Geometry: final body of the model. Coordinates: model frame, mm. Give positions to 0.01 mm unless a question says otherwise; leave off trailing zeros. Loops run counter-clockwise (first coordinate to the right, second up) from the corner with the lowest first, then second, coordinate; pieces in that order, holes last. Notation, with made-up numbers: (13, 65.25) - (55, 65.25) arc R25 ccw to (55, 87.25) - close; hole circle Ø7 at (-1, 60). An arc over 180 degrees is marked (long way). Answer in a Markdown table with one row per item.
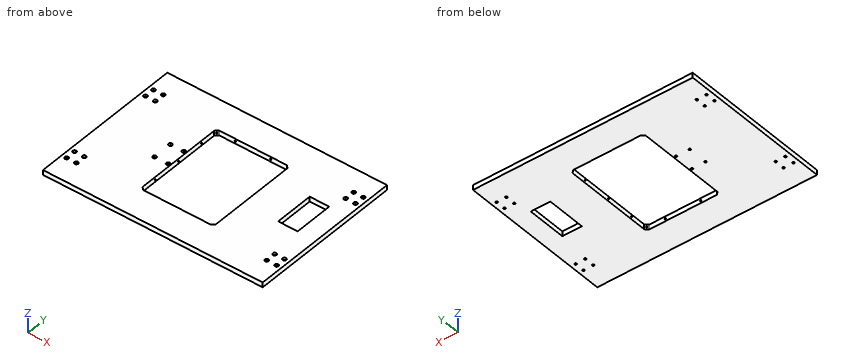
from build123d import *

# Parameters (mm, degrees)
SKETCH1_W                                            = 900
SKETCH1_H                                            = 630
BOSS_EXTRUDE1_DEPTH                                  = 20
SKETCH2_W                                            = 300
SKETCH2_H                                            = 385
CUT_EXTRUDE1_DEPTH                                   = 550.65898519
CHAMFER1_SIZE                                        = 11
FILLET1_R                                            = 3
M6_TAPPED_HOLE2_AT_2_COUNT                           = 2
M6_TAPPED_HOLE2_AT_2_PITCH                           = 117.5
CBORE_FOR_M8_HEXAGON_SOCKET_HEAD_CAP_SCR_D           = 8.4
CBORE_FOR_M8_HEXAGON_SOCKET_HEAD_CAP_SCR_CBORE_D     = 15
CBORE_FOR_M8_HEXAGON_SOCKET_HEAD_CAP_SCR_CBORE_DEPTH = 9
SKETCH13_W                                           = 80
SKETCH13_H                                           = 160
CUT_EXTRUDE3_DEPTH                                   = 550.65898519


with BuildPart() as part:
    # Sketch1 → Boss-Extrude1 (new body)
    with BuildSketch(Plane.XY):
        Rectangle(SKETCH1_W, SKETCH1_H)
    extrude(amount=BOSS_EXTRUDE1_DEPTH)

    # Sketch2 → Cut-Extrude1 (cut, through all)
    with BuildSketch(Plane.XY.offset(20)):
        Rectangle(SKETCH2_W, SKETCH2_H)
    extrude(amount=-CUT_EXTRUDE1_DEPTH, mode=Mode.SUBTRACT)

    # Chamfer1
    chamfer1_edges = [part.edges().sort_by_distance(p)[0] for p in [
        (-150, -192.5, 10),
        (-150, 192.5, 10),
        (150, 192.5, 10),
        (150, -192.5, 10),
    ]]
    chamfer(chamfer1_edges, length=CHAMFER1_SIZE)

    # Sketch4 → M6 Tapped Hole1 (revolve, cut)
    with BuildSketch(Plane(origin=(-144.5, 187, 10), x_dir=(0.7071067811865441, 0.7071067811865509, 0), z_dir=(0, 0, 1))):
        Polygon((0, 0), (0, 31.502151548), (2.5, 30), (2.5, 0), align=None)
    m6_tapped_hole1 = revolve(axis=Axis((-140.009871939, 182.509871939, 10), (-0.7071067811865509, 0.7071067811865442, 0)), mode=Mode.SUBTRACT)

    # Fillet1
    fillet1_edges = [part.edges().sort_by_distance(p)[0] for p in [
        (139, -192.5, 10),
        (-139, -192.5, 10),
        (-150, 181.5, 10),
        (-150, -181.5, 10),
        (150, 181.5, 10),
        (150, -181.5, 10),
        (-139, 192.5, 10),
        (139, 192.5, 10),
    ]]
    fillet(fillet1_edges, radius=FILLET1_R)

    # Sketch6 → M6 Tapped Hole2 (revolve, cut)
    with BuildSketch(Plane(origin=(-150, 0, 10), x_dir=(0, 0, -1), z_dir=(0, 1, 0))):
        Polygon((0, 0), (0, 31.502151548), (2.5, 30), (2.5, 0), align=None)
    m6_tapped_hole2 = revolve(axis=Axis((-143.65, 0, 10), (-1, 0, 0)), mode=Mode.SUBTRACT)

    # M6 Tapped Hole2 at 2: M6 Tapped Hole2 ×2
    with Locations(*[(0, i * M6_TAPPED_HOLE2_AT_2_PITCH, 0) for i in range(1, M6_TAPPED_HOLE2_AT_2_COUNT)]):
        add(m6_tapped_hole2, mode=Mode.SUBTRACT)

    # Sketch8 → M6 Tapped Hole3 (revolve, cut)
    with BuildSketch(Plane(origin=(-72.5, 192.5, 10), x_dir=(0, 0, -1), z_dir=(1, 0, 0))):
        Polygon((0, 0), (0, 31.502151548), (2.5, 30), (2.5, 0), align=None)
    m6_tapped_hole3 = revolve(axis=Axis((-72.5, 186.15, 10), (0, 1, 0)), mode=Mode.SUBTRACT)

    # Mirror1: M6 Tapped Hole1, M6 Tapped Hole2, M6 Tapped Hole3 across plane
    add(m6_tapped_hole1.mirror(Plane(origin=(0, 0, 0), x_dir=(0, 0, 1), z_dir=(1, 0, 0))), mode=Mode.SUBTRACT)
    add(m6_tapped_hole2.mirror(Plane(origin=(0, 0, 0), x_dir=(0, 0, 1), z_dir=(1, 0, 0))), mode=Mode.SUBTRACT)
    add(m6_tapped_hole3.mirror(Plane(origin=(0, 0, 0), x_dir=(0, 0, 1), z_dir=(1, 0, 0))), mode=Mode.SUBTRACT)

    # Mirror1 copy 1 sketch → Mirror1 copy 1 (revolve, cut)
    with BuildSketch(Plane(origin=(150, 117.5, 10), x_dir=(0, 0, -1), z_dir=(0, 1, 0))):
        Polygon((0, 0), (0, -31.502151548), (2.5, -30), (2.5, 0), align=None)
    revolve(axis=Axis((143.65, 117.5, 10), (-1, 0, 0)), mode=Mode.SUBTRACT)

    # Mirror1 at the second plane: M6 Tapped Hole1, M6 Tapped Hole2, M6 Tapped Hole3 across plane
    add(m6_tapped_hole1.mirror(Plane.ZX), mode=Mode.SUBTRACT)
    add(m6_tapped_hole2.mirror(Plane.ZX), mode=Mode.SUBTRACT)
    add(m6_tapped_hole3.mirror(Plane.ZX), mode=Mode.SUBTRACT)

    # Mirror1 at the second plane copy 1 sketc → Mirror1 at the second plane copy 1 (revolve, cut)
    with BuildSketch(Plane(origin=(-150, -117.5, 10), x_dir=(0, 0, -1), z_dir=(0, -1, 0))):
        Polygon((0, 0), (0, -31.502151548), (2.5, -30), (2.5, 0), align=None)
    revolve(axis=Axis((-143.65, -117.5, 10), (1, 0, 0)), mode=Mode.SUBTRACT)

    # Mirror1 at the second plane copy 2 sketc → Mirror1 at the second plane copy 2 (revolve, cut)
    with BuildSketch(Plane(origin=(144.5, -187, 10), x_dir=(-0.7071067811865441, -0.7071067811865509, 0), z_dir=(0, 0, 1))):
        Polygon((0, 0), (0, 31.502151548), (2.5, 30), (2.5, 0), align=None)
    revolve(axis=Axis((140.009871939, -182.509871939, 10), (0.7071067811865509, -0.7071067811865442, 0)), mode=Mode.SUBTRACT)

    # Mirror1 at the second plane copy 3 sketc → Mirror1 at the second plane copy 3 (revolve, cut)
    with BuildSketch(Plane(origin=(150, 0, 10), x_dir=(0, 0, -1), z_dir=(0, -1, 0))):
        Polygon((0, 0), (0, 31.502151548), (2.5, 30), (2.5, 0), align=None)
    revolve(axis=Axis((143.65, 0, 10), (1, 0, 0)), mode=Mode.SUBTRACT)

    # Mirror1 at the second plane copy 4 sketc → Mirror1 at the second plane copy 4 (revolve, cut)
    with BuildSketch(Plane(origin=(72.5, -192.5, 10), x_dir=(0, 0, -1), z_dir=(-1, 0, 0))):
        Polygon((0, 0), (0, 31.502151548), (2.5, 30), (2.5, 0), align=None)
    revolve(axis=Axis((72.5, -186.15, 10), (0, -1, 0)), mode=Mode.SUBTRACT)

    # Mirror1 at the second plane copy 5 sketc → Mirror1 at the second plane copy 5 (revolve, cut)
    with BuildSketch(Plane(origin=(150, -117.5, 10), x_dir=(0, 0, -1), z_dir=(0, -1, 0))):
        Polygon((0, 0), (0, 31.502151548), (2.5, 30), (2.5, 0), align=None)
    revolve(axis=Axis((143.65, -117.5, 10), (1, 0, 0)), mode=Mode.SUBTRACT)

    # CBORE for M8 Hexagon socket head cap screws1 (through all)
    with Locations(Plane.XY.offset(20)):
        with Locations((-430, 220), (-390, 220), (-430, 180), (-390, 180), (-215.00186624, 40), (-160.00186624, 40), (390, 220), (430, 220), (390, 180), (430, 180), (430, -180), (390, -180), (430, -220), (390, -220), (-160.00186624, -40), (-215.00186624, -40), (-390, -180), (-430, -180), (-390, -220), (-430, -220)):
            CounterBoreHole(CBORE_FOR_M8_HEXAGON_SOCKET_HEAD_CAP_SCR_D / 2, CBORE_FOR_M8_HEXAGON_SOCKET_HEAD_CAP_SCR_CBORE_D / 2, CBORE_FOR_M8_HEXAGON_SOCKET_HEAD_CAP_SCR_CBORE_DEPTH)

    # Sketch13 → Cut-Extrude3 (cut, through all)
    with BuildSketch(Plane.XY.offset(20)):
        with Locations((335, 35)):
            Rectangle(SKETCH13_W, SKETCH13_H)
    extrude(amount=-CUT_EXTRUDE3_DEPTH, mode=Mode.SUBTRACT)


solid = part.part
Q1. Material intervals for line 1 along X through (y, z) = (92, 8.5); line 2 along Y through (x, z) = (-430, 13.5); line 3 along Y through (x, z) = (-430, 2.75), sorted ascending.
Check values:
| item | result |
|---|---|
| line 1 | -450 to -150, 150 to 295, 375 to 450 |
| line 2 | -315 to -227.5, -212.5 to -187.5, -172.5 to 172.5, 187.5 to 212.5, 227.5 to 315 |
| line 3 | -315 to -224.2, -215.8 to -184.2, -175.8 to 175.8, 184.2 to 215.8, 224.2 to 315 |
Q2. First-contact query: pin 1 (11 mm diameter, centred on x = 390, y = -220, fed in from +Z); pin 2 (7.5 mm diameter, centred on x = -430, y = 220, fed in from +Z); pin 3 (16.5 mm diameter, centred on x = -430, y = -222, fed in from +Z). Flat tips, straight axial feed; report the tip coordinate or a pass-through.
Check values:
| item | result |
|---|---|
| pin 1 | z = 11 |
| pin 2 | through |
| pin 3 | z = 20 |
Q3. Cut plane A-A (x = -20). Output: boundary loops of the cut face in (y, z), and give its area (3 significant figures).
Check values:
| item | result |
|---|---|
| outline | (-315, 0) - (-192.5, 0) - (-192.5, 20) - (-315, 20) - close; (192.5, 0) - (315, 0) - (315, 20) - (192.5, 20) - close |
| area | 4,900 mm² |
Q4. Cut plane B-B (y = 88). Output: boundary loops of the cut face in (x, z).
Check values:
| item | result |
|---|---|
| outline | (-450, 0) - (-150, 0) - (-150, 20) - (-450, 20) - close; (150, 0) - (295, 0) - (295, 20) - (150, 20) - close; (375, 0) - (450, 0) - (450, 20) - (375, 20) - close |
